Can you work these out from the model? Positions are in its coordinate system, mm. A direction names the side the tool comes from. Round coordinates to 2 decimals unless told otherwise and drop trailing zeros. Loops run counter-clockwise (first coordinate to the right, second up) from the corner with the lowest first, then second, coordinate; pieces in that order, holes last. Notation, with made-up numbers: (56.25, -11.5) - (99.25, -11.5) arc R33 ccw to (99.25, 21.5) - close; hole circle Ø6 at (-15, 19). An arc over 180 degrees is marked (long way). Answer as CSV lines item,"result".
```python
from build123d import *

# Parameters (mm, degrees)
SKETCH1_W           = 30
SKETCH1_H           = 60
BOSS_EXTRUDE1_DEPTH = 50
BOSS_EXTRUDE2_DEPTH = 90
SKETCH3_R           = 7.5
CUT_EXTRUDE1_DEPTH  = 90
CUT_EXTRUDE2_DEPTH  = 90
SKETCH5_W           = 16.87997937
SKETCH5_H           = 20
BOSS_EXTRUDE3_DEPTH = 20
CUT_EXTRUDE3_DEPTH  = 20
CUT_EXTRUDE4_DEPTH  = 10
SKETCH8_W           = 10
SKETCH8_H           = 44.983560701
CUT_EXTRUDE5_DEPTH  = 50


with BuildPart() as part:
    # Sketch1 → Boss-Extrude1 (new body)
    with BuildSketch(Plane(origin=(0, 0, 0), x_dir=(1, 0, 0), z_dir=(0, 1, 0))):
        with Locations((-15, -21.017964072)):
            Rectangle(SKETCH1_W, SKETCH1_H)
    extrude(amount=-BOSS_EXTRUDE1_DEPTH)

    # Sketch2 → Boss-Extrude2 (add)
    with BuildSketch(Plane(origin=(0, 0, 0), x_dir=(0, 0, -1), z_dir=(1, 0, 0))):
        Polygon((-21.017964072, -50), (-41.017964072, -50), (-41.017964072, -20), (-1.017964072, -20), (-1.017964072, -50), align=None)
    extrude(amount=BOSS_EXTRUDE2_DEPTH)

    # Sketch3 → Cut-Extrude1 (cut)
    with BuildSketch(Plane.XY.offset(41.017964072)):
        with Locations((35.036901586, -35)):
            Circle(SKETCH3_R)
    extrude(amount=-CUT_EXTRUDE1_DEPTH, mode=Mode.SUBTRACT)

    # Sketch4 → Cut-Extrude2 (cut)
    with BuildSketch(Plane(origin=(0, -20, 0), x_dir=(1, 0, 0), z_dir=(0, 1, 0))):
        Polygon((70, -1.017964072), (90, -13.353113833), (90, -1.017964072), align=None)
        Polygon((70, -41.017964072), (90, -30.233093203), (90, -41.017964072), align=None)
    extrude(amount=-CUT_EXTRUDE2_DEPTH, mode=Mode.SUBTRACT)

    # Sketch5 → Boss-Extrude3 (add)
    with BuildSketch(Plane(origin=(90, 0, 0), x_dir=(0, 0, -1), z_dir=(1, 0, 0))):
        with Locations((-21.793103518, -40)):
            Rectangle(SKETCH5_W, SKETCH5_H)
    extrude(amount=BOSS_EXTRUDE3_DEPTH)

    # Sketch6 → Cut-Extrude3 (cut)
    with BuildSketch(Plane(origin=(0, -30, 0), x_dir=(1, 0, 0), z_dir=(0, 1, 0))):
        Polygon((110, -13.353113833), (90, -13.353113833), (110, -21.793103518), align=None)
        Polygon((110, -30.233093203), (110, -21.793103518), (90, -30.233093203), align=None)
    extrude(amount=-CUT_EXTRUDE3_DEPTH, mode=Mode.SUBTRACT)

    # Sketch7 → Cut-Extrude4 (cut)
    with BuildSketch(Plane(origin=(0, 0, 0), x_dir=(1, 0, 0), z_dir=(0, 1, 0))):
        Polygon((-30, 1.482035928), (-30, -43.501524773), (-20, -43.501524773), (-20, -33.517964072), (0, -33.517964072), (0, -8.517964072), (-20, -8.517964072), (-20, 1.482035928), align=None)
    extrude(amount=-CUT_EXTRUDE4_DEPTH, mode=Mode.SUBTRACT)

    # Sketch8 → Cut-Extrude5 (cut)
    with BuildSketch(Plane(origin=(0, -10, 0), x_dir=(1, 0, 0), z_dir=(0, 1, 0))):
        with Locations((-25, -21.009744422)):
            Rectangle(SKETCH8_W, SKETCH8_H)
    extrude(amount=-CUT_EXTRUDE5_DEPTH, mode=Mode.SUBTRACT)


solid = part.part
```
Q1. Imagine slicing it at B-B (x = 33). Write out the boundary of the cut face in (y, z), then the cut area to 3 significant figures.
Checks:
outline,"(-50, 1.02) - (-42.22, 1.02) - (-42.22, 41.02) - (-50, 41.02) - close; (-27.78, 1.02) - (-20, 1.02) - (-20, 41.02) - (-27.78, 41.02) - close"
area,"623 mm²"
Q2. Imagine slicing it at C-C (z = 6). Write out the boundary of the cut face in (x, y).
Checks:
outline,"(-20, -50) - (78.08, -50) - (78.08, -20) - (0, -20) - (0, 0) - (-20, 0) - close; hole circle Ø15 at (35.04, -35)"
Q3. Imagine slicing it at D-D (y = -13.5). Write out the boundary of the cut face in (x, z).
Checks:
outline,"(-30, -8.98) - (0, -8.98) - (0, 51.02) - (-30, 51.02) - (-30, 43.5) - (-20, 43.5) - (-20, -1.48) - (-30, -1.48) - close"
Q4. I'm going to push flat-ended pins straight in: pin 1 Ø1 at (x, z) = (-8.5, 14) entering from +Y; pin 2 Ø8 at (y, z) = (-13, 8.5) entering from -X; pin 3 Ø8 at (y, z) = (-8, 35.5) entering from +X. Where does each tip first touch, or does it pass through?
Checks:
pin 1,"y = -10"
pin 2,"x = -20"
pin 3,"x = 0"
Q5. We'd pull the mould along Z, two halves only. Please class faces 6 (the flat face through (0, -19, 21)), 7 (the flat face through (79.86, -34.79, 35.7)), 8 (the flat face through (-25, -25, 43.502)), 9 (the flat face through (-15, -25, -8.982)): pulls with the +Z half, pulls with the -Z half, needs draft (parallel to the pull), parting line crosses it, or undercut.
Checks:
face 6,"needs draft"
face 7,"pulls with the +Z half"
face 8,"undercut"
face 9,"pulls with the -Z half"
Q6. If I drill on line 1 along X through (y, z) = (-39, 42.5); line 2 along Y through (x, z) = (53, 4.5); line 3 along X through (y, z) = (-35.5, -5.5), over which ranges is the centre line in solid material (lowest first)? Write a range as [from, to].
Checks:
line 1,"[-20, 0]"
line 2,"[-50, -20]"
line 3,"[-30, 0]"
Q7. Imagine slicing it at A-A (y = -35). Write out the boundary of the cut face in (x, z), then the cut area to 3 significant figures.
Checks:
outline,"(-30, -8.98) - (0, -8.98) - (0, 1.02) - (27.54, 1.02) - (27.54, 41.02) - (0, 41.02) - (0, 51.02) - (-30, 51.02) - (-30, 43.5) - (-20, 43.5) - (-20, -1.48) - (-30, -1.48) - close; (42.54, 1.02) - (70, 1.02) - (90, 13.35) - (110, 21.79) - (90, 30.23) - (70, 41.02) - (42.54, 41.02) - close"
area,"4,290 mm²"
Q8. On a 3-axis mill with a long thin cutter (end or side, diameter ignored), from which of +Z, -Z, +X, -X, +Y, -Y can I reach the whole of each face in a straight line? I mean faces 1 (the flat face through (-20, -25, 21)), 2 (the flat face through (27, -35, 1.018)), 3 (the flat face through (-10, -5, 33.518)), 4 (the flat face through (44, -20, 21)), 5 (the flat face through (27, -35, 41.018)). Say none if no direction works.
Checks:
face 1,"-X, +Y, -Y"
face 2,"-Z, +X, +Y, -Y"
face 3,"+X, -X, +Y"
face 4,"+Z, -Z, +X, +Y"
face 5,"+Z, +X, +Y, -Y"
